Verification items for the finished model (mm, model axes). A direction names the side the tool comes from. Give positions to 0.01 mm unless a question says otherwise; leave off trailing zeros. Order: outer loops, then holes, each group sorted by start corner. A loop starts at its lowest first (then second) coordinate and runs counter-clockwise, first axis right, second up.
(1) Sectioned sample at A-A on z = 12.5. Record the cut outline in (x, y).
(2) Sectioned sample at B-B on x = 0. Record the cut outline in (y, z), plus the area to 3 significant figures.
(3) Mould release check, pull along Y, two halves, no side actions. Record for faces 4 (the face through (0, -0.25, 8)), 5 (the face through (-0.1, -3.1, 14)), 6 (the face through (0, 2.3, 15.3)): pulls with the +Y half, pulls with the -Y half, needs draft (parallel to the pull), parting line crosses it, or undercut.
(4) Access from +Z, -Z, +X, -X, +Y, -Y to the whole of each face (thin tool, end or side, straight path). Record for faces 1 (the face through (-0.1, -2.9, 6.7)), 2 (the face through (0, 0, 0)), 3 (the face through (0.1, 3.1, 14)).
(5) Gauge pin test, flat ends, axial feed: pin 1 (3 mm diameter, centred on x = -1.5, z = 5.5, fed in from -Y); pin 2 (1.5 mm diameter, centred on x = -2.5, z = 9.5, fed in from +Y); pin 3 (1.9 mm diameter, centred on x = 1, z = 7.5, fed in from +Y). Record the tip position at first contact, or that the pin passes through.
(6) Sectioned sample at C-C on y = -3.5. Record the cut outline in (x, z).
(7) Scan lines: L1, parallel to Y at x = 0, z = 11.5; L2, parallel to Z at x = 0.25, y = 3.5; L3, parallel to X at y = -2, z = 7.5. Record each from-to range of solid material in increasing order.
```python
from build123d import *

# Parameters (mm, degrees)
F1_DEPTH = 1.9
F2_DEPTH = 13.5
F4_DEPTH = 2
F5_SIZE  = 1


with BuildPart() as f1:
    # F0 (on Top) → F1 (new body)
    with BuildSketch(Plane.XY):
        with BuildLine():
            Line((2.8892040426, 0.25), (4.2927264064, 0.25))
            ThreePointArc((4.2927264064, 0.25), (0, 4.3), (-4.2927264064, 0.25))
            Line((-4.2927264064, 0.25), (-2.8892040426, 0.25))
            ThreePointArc((-2.8892040426, 0.25), (0, 2.9), (2.8892040426, 0.25))
        make_face()
        with BuildLine():
            Line((0, 0.25), (2.8892040426, 0.25))
            ThreePointArc((2.8892040426, 0.25), (0, 2.9), (-2.8892040426, 0.25))
            Line((-2.8892040426, 0.25), (0, 0.25))
        make_face()
        with BuildLine():
            Line((-2.8892040426, 0.25), (-4.2927264064, 0.25))
            ThreePointArc((-4.2927264064, 0.25), (-4.3, 0), (-4.2927264064, -0.25))
            Line((-4.2927264064, -0.25), (-2.8892040426, -0.25))
            ThreePointArc((-2.8892040426, -0.25), (-2.9, 0), (-2.8892040426, 0.25))
        make_face()
        with BuildLine():
            ThreePointArc((4.2927264064, -0.25), (4.2981812169, -0.125052894), (4.3, 0))
            ThreePointArc((4.3, 0), (4.2981812169, 0.125052894), (4.2927264064, 0.25))
            Line((4.2927264064, 0.25), (2.8892040426, 0.25))
            ThreePointArc((2.8892040426, 0.25), (2.8972997535, 0.1251164984), (2.9, 0))
            ThreePointArc((2.9, 0), (2.8972997535, -0.1251164984), (2.8892040426, -0.25))
            Line((2.8892040426, -0.25), (4.2927264064, -0.25))
        make_face()
        with BuildLine():
            ThreePointArc((-4.2927264064, -0.25), (0, -4.3), (4.2927264064, -0.25))
            Line((4.2927264064, -0.25), (2.8892040426, -0.25))
            ThreePointArc((2.8892040426, -0.25), (0, -2.9), (-2.8892040426, -0.25))
            Line((-2.8892040426, -0.25), (-4.2927264064, -0.25))
        make_face()
        with BuildLine():
            ThreePointArc((-2.8892040426, -0.25), (0, -2.9), (2.8892040426, -0.25))
            Line((2.8892040426, -0.25), (0, -0.25))
            Line((0, -0.25), (-2.8892040426, -0.25))
        make_face()
        with BuildLine():
            ThreePointArc((2.9, 0), (2.8972997535, 0.1251164984), (2.8892040426, 0.25))
            Line((2.8892040426, 0.25), (0, 0.25))
            Line((0, 0.25), (-2.8892040426, 0.25))
            ThreePointArc((-2.8892040426, 0.25), (-2.9, 0), (-2.8892040426, -0.25))
            Line((-2.8892040426, -0.25), (0, -0.25))
            Line((0, -0.25), (2.8892040426, -0.25))
            ThreePointArc((2.8892040426, -0.25), (2.8972997535, -0.1251164984), (2.9, 0))
        make_face()
    extrude(amount=-F1_DEPTH)

    # F0 (on Top) → F2 (join)
    with BuildSketch(Plane.XY):
        with BuildLine():
            ThreePointArc((-2.8892040426, -0.25), (0, -2.9), (2.8892040426, -0.25))
            Line((2.8892040426, -0.25), (0, -0.25))
            Line((0, -0.25), (-2.8892040426, -0.25))
        make_face()
        with BuildLine():
            Line((0, 0.25), (2.8892040426, 0.25))
            ThreePointArc((2.8892040426, 0.25), (0, 2.9), (-2.8892040426, 0.25))
            Line((-2.8892040426, 0.25), (0, 0.25))
        make_face()
    extrude(amount=F2_DEPTH)

    # F3 (on face) → F4 (join)
    with BuildSketch(Plane.XY.offset(13.5)):
        with BuildLine():
            ThreePointArc((-3.0899029111, -0.25), (0, -3.1), (3.0899029111, -0.25))
            Line((3.0899029111, -0.25), (0, -0.25))
            Line((0, -0.25), (-3.0899029111, -0.25))
        make_face()
        with BuildLine():
            Line((0, 0.25), (2.8892040426, 0.25))
            ThreePointArc((2.8892040426, 0.25), (0, 2.9), (-2.8892040426, 0.25))
            Line((-2.8892040426, 0.25), (0, 0.25))
        make_face()
        with BuildLine():
            Line((2.8892040426, 0.25), (3.0899029111, 0.25))
            ThreePointArc((3.0899029111, 0.25), (0, 3.1), (-3.0899029111, 0.25))
            Line((-3.0899029111, 0.25), (-2.8892040426, 0.25))
            ThreePointArc((-2.8892040426, 0.25), (0, 2.9), (2.8892040426, 0.25))
        make_face()
    extrude(amount=F4_DEPTH)

    # F5
    f5_edges = [f1.edges().sort_by_distance(p)[0] for p in [
        (0, 3.1, 15.5),
        (0, -3.1, 15.5),
    ]]
    chamfer(f5_edges, length=F5_SIZE)


solid = f1.part
```
Ans:
1. outline: (-2.89, -0.25) arc R2.9 ccw to (2.89, -0.25) - close; (-2.89, 0.25) - (2.89, 0.25) arc R2.9 ccw to start
2. outline: (-4.3, -1.9) - (4.3, -1.9) - (4.3, 0) - (2.9, 0) - (2.9, 13.5) - (3.1, 13.5) - (3.1, 14.5) - (2.1, 15.5) - (0.25, 15.5) - (0.25, 0) - (-0.25, 0) - (-0.25, 15.5) - (-2.1, 15.5) - (-3.1, 14.5) - (-3.1, 13.5) - (-2.9, 13.5) - (-2.9, 0) - (-4.3, 0) - close
2. area: 98.3 mm2
3. face 4: undercut
3. face 5: pulls with the -Y half
3. face 6: pulls with the +Y half
4. face 1: -Y
4. face 2: none
4. face 3: +Z, +Y
5. pin 1: stops at y = -2.9
5. pin 2: stops at y = 2.31
5. pin 3: stops at y = 2.9
6. outline: (-2.5, -1.9) - (2.5, -1.9) - (2.5, 0) - (-2.5, 0) - close
7. L1: y = -2.9 to -0.25, 0.25 to 2.9
7. L2: z = -1.9 to 0
7. L3: x = -2.1 to 2.1
